```python
from build123d import *

# Parameters (mm, degrees)
SKETCH1_W                   = 25.4
SKETCH1_H                   = 25.4
BOSS_EXTRUDE1_DEPTH         = 25.4
F_1_4_0_25_DIAMETER_HOLE1_D = 6.35
F_1_4_0_25_DIAMETER_HOLE2_D = 6.35
F_1_4_0_25_DIAMETER_HOLE3_D = 6.35


with BuildPart() as part:
    # Sketch1 → Boss-Extrude1 (new body)
    with BuildSketch(Plane.XY):
        Rectangle(SKETCH1_W, SKETCH1_H)
    extrude(amount=BOSS_EXTRUDE1_DEPTH)

    # 1/4 (0.25) Diameter Hole1 (through all)
    with Locations(Plane(origin=(0, 0, 0), x_dir=(-1, 0, 0), z_dir=(0, 0, -1))):
        with Locations((0, 0)):
            Hole(F_1_4_0_25_DIAMETER_HOLE1_D / 2)

    # 1/4 (0.25) Diameter Hole2 (through all)
    with Locations(Plane(origin=(0, 12.7, 0), x_dir=(1, 0, 0), z_dir=(0, 1, 0))):
        with Locations((0, -12.7)):
            Hole(F_1_4_0_25_DIAMETER_HOLE2_D / 2)

    # 1/4 (0.25) Diameter Hole3 (through all)
    with Locations(Plane.ZY.offset(12.7)):
        with Locations((12.7, 0)):
            Hole(F_1_4_0_25_DIAMETER_HOLE3_D / 2)


solid = part.part
```
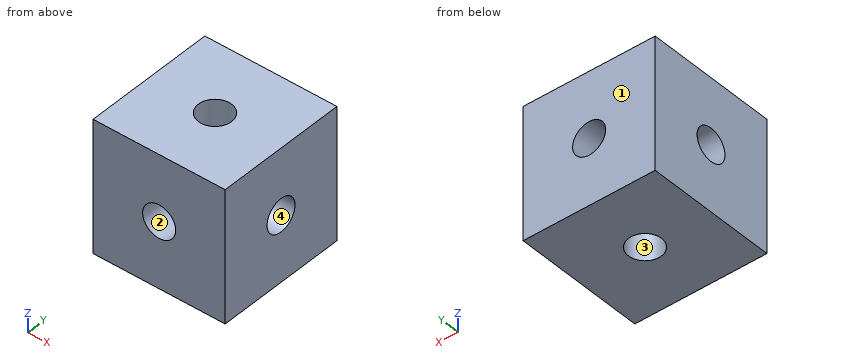
Input: part model. Units: mm. Frame: model coordinates. Face numbers are marked on the shaded views. Give positions to 0.01 mm unless a question says otherwise; leave off trailing zeros. Write each loop counter-clockwise with the first axis right and the second up, starting at its lowest first coordinate (ties: lowest second). Pieces come first, ordered by that corner, then holes. Notation, with made-up numbers: (-26.75, 68.25) - (-19.75, 68.25) arc R7 cw to (-19.75, 81.25) - close; hole circle Ø2 at (44, -5). An arc over 180 degrees is marked (long way). Write item = value, one per line. Start each with the question number.
1) Cut plane C-C (x = -4.5). Return loops of the section in (y, z) (3 decimals).
2) Material intervals for L1, parallel to Z at x = 6.25, y = 0 (3 decimals); L2, parallel to X at y = -8.25, z = 12.7 (3 decimals), sorted ascending. Write a range as [from, to].
3) Cut plane B-B (y = 0). Return loops of the section in (x, z) (3 decimals).
4) Cut plane A-A (z = 12.7). Return loops of the section in (x, y) (3 decimals).
5) Cut plane D-D (z = 2.25). Return loops of the section in (x, y) (3 decimals), and give its area (3 significant figures).
6) Draft query along Y for the marked faces 1, 2, 3 and 4. Return one class per face: pulls with the +Y half, pulls with the -Y half, needs draft (parallel to the pull), parting line crosses it, or undercut.
Answers follow:
q1.outline = (-12.7, 0) - (12.7, 0) - (12.7, 25.4) - (-12.7, 25.4) - close; hole circle Ø6.35 at (0, 12.7)
q2.L1 = [0, 9.525], [15.875, 25.4]
q2.L2 = [-12.7, -3.175], [3.175, 12.7]
q3.outline = (-12.7, 0) - (-3.175, 0) - (-3.175, 9.525) - (-12.7, 9.525) - close; (-12.7, 15.875) - (-3.175, 15.875) - (-3.175, 25.4) - (-12.7, 25.4) - close; (3.175, 0) - (12.7, 0) - (12.7, 9.525) - (3.175, 9.525) - close; (3.175, 15.875) - (12.7, 15.875) - (12.7, 25.4) - (3.175, 25.4) - close
q4.outline = (-12.7, -12.7) - (-3.175, -12.7) - (-3.175, -3.175) - (-12.7, -3.175) - close; (-12.7, 3.175) - (-3.175, 3.175) - (-3.175, 12.7) - (-12.7, 12.7) - close; (3.175, -12.7) - (12.7, -12.7) - (12.7, -3.175) - (3.175, -3.175) - close; (3.175, 3.175) - (12.7, 3.175) - (12.7, 12.7) - (3.175, 12.7) - close
q5.outline = (-12.7, -12.7) - (12.7, -12.7) - (12.7, 12.7) - (-12.7, 12.7) - close; hole circle Ø6.35 at (0, 0)
q5.area = 613 mm^2
q6.face_1 = pulls with the +Y half
q6.face_2 = needs draft
q6.face_3 = undercut
q6.face_4 = undercut
